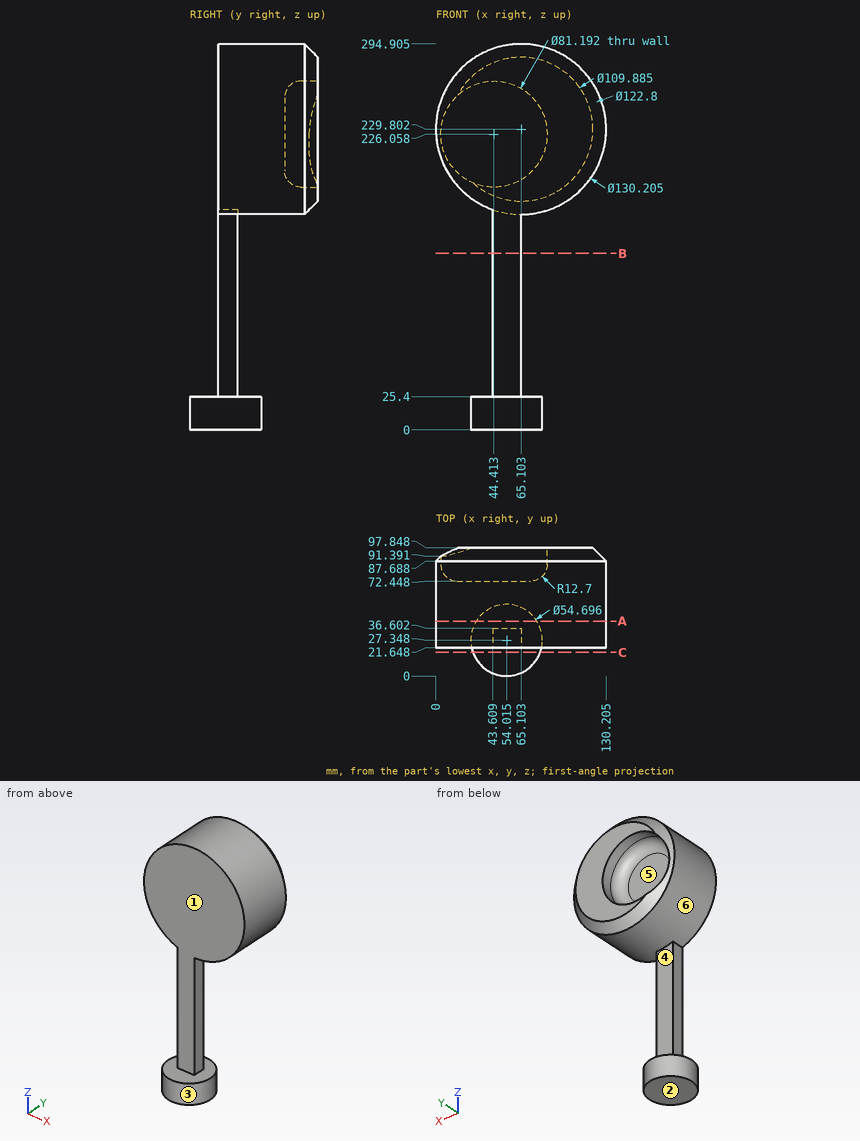
Print and shaded views of the part. All mm, measured from the part's lowest x, y and z. A direction names the side the tool comes from. Coordinates: 2 decimals unless noted, no trailing zeros. Order: outer loops, then holes, each group sorted by start corner. A loop starts at its lowest first (then second) coordinate and runs counter-clockwise, first axis right, second up.
(1) Slice it at B-B, the plane z = 135. Write the cut outline in (x, y), and give its area (3 significant figures).
Check sheet entries:
outline: (43.61, 21.65) - (65.1, 21.65) - (65.1, 36.6) - (43.61, 36.6) - close
area: 321 mm2
(2) Tool access for the marked faces 1, 2 and 3: list every direction of +Z, -Z, +X, -X, +Y, -Y with a clear straight run to the whole face (end or side of a thin tool).
Check sheet entries:
face 1: +Z, +X, -X, -Y
face 2: -Z, +X, -X, +Y, -Y
face 3: -Z
(3) Probe L1, parallel to Z at x = 61.5, y = 6; L2, parallel to X at y = 34.5, z = 75; L3, parallel to Y at x = 26.5, z = 233. List the from-to ranges inside material, lowest first.
Check sheet entries:
L1: z = 0 to 25.4
L2: x = 43.61 to 65.1
L3: y = 21.65 to 72.45
(4) Pin check, flat tips, straight feed: pin 1 Ø4 at (x, z) = (16.5, 191) entering from +Y; pin 2 Ø1.5 at (x, z) = (46.5, 112) entering from +Y; pin 3 Ø16.5 at (x, y) = (47, 15.5) entering from +Z. Stop position of each tip, or through.
Check sheet entries:
pin 1: stops at y = 92.6
pin 2: stops at y = 36.6
pin 3: stops at z = 293.67
(5) Pull direction X, two halves, no side cores. Call the marked faces 4, 5 and 6: pulls with the +X half, pulls with the -X half, needs draft (parallel to the pull), parting line crosses it, or undercut.
Check sheet entries:
face 4: needs draft
face 5: undercut
face 6: parting line crosses it
(6) Slice it at A-A, the plane y = 42. Write the cut outline in (x, z) (1 decimal), and give its area (3 significant figures).
Check sheet entries:
outline: circle Ø130.2 at (65.1, 229.8); (30.9, 0) - (77.1, 0) - (77.1, 25.4) - (30.9, 25.4) - close
area: 14,500 mm2
(7) Slice it at C-C, the plane y = 18. Write the cut outline in (x, z) (1 decimal).
Check sheet entries:
outline: (28.3, 0) - (79.7, 0) - (79.7, 25.4) - (28.3, 25.4) - close
